Read the model definition and answer for the solid it produces. Units are mm, in the model's axes. Face numbers are marked on the shaded views. A direction names the side the tool comes from. Round coordinates to 2 decimals unless told otherwise and drop trailing zeros. Order: outer loops, then holes, each group sorted by start corner. A loop starts at its lowest first (then second) coordinate and runs counter-clockwise, first axis right, second up. Notation, with made-up numbers: (-31.75, -5.75) -> (27.25, -5.75) arc R29 cw to (27.25, 24.25) -> close; hole circle Ø8 at (17, -8). An arc over 180 degrees is marked (long way). Use a Markdown table: item, result. Add a question column.
1. Section B-B, the plane x = 5 is taken. Give the vertices of the cut face in (y, z).
2. The mould has two halves that part along Y. Classify the marked faces 3, 4, 5 and 6: +Y half, -Y half, draft (parallel to the pull), parting line (faces both ways), or undercut.
3. For the marked faces 1 and 2, determine the directions among +Z, -Z, +X, -X, +Y, -Y from which every point of the face is accessible in a straight line to the end or side of a thin tool.
4. Given pin 1 (5 mm diameter, centred on x = 25, y = -5, fed in from -Z), flat-ended and moving along its own axis, determine where the tip first touches the part or whether it passes through.
5. Section C-C, the plane z = 2.55 is taken. Give the vertices of the cut face in (x, y).
6. Section D-D, the plane y = -30.5 is taken. Give the vertices of the cut face in (x, z).
7. Consider L1, parallel to Y at x = 25, z = 1.5; L2, parallel to X at y = -26.5, z = 2.35; L3, parallel to Y at x = 11, z = 0.3. Determine where each line is inside the solid, lowest interval first. Write a range as [from, to].
8. Section A-A, the plane y = -5 is taken. Give the vertices of the cut face in (x, z), then the cut area to 3 significant figures.
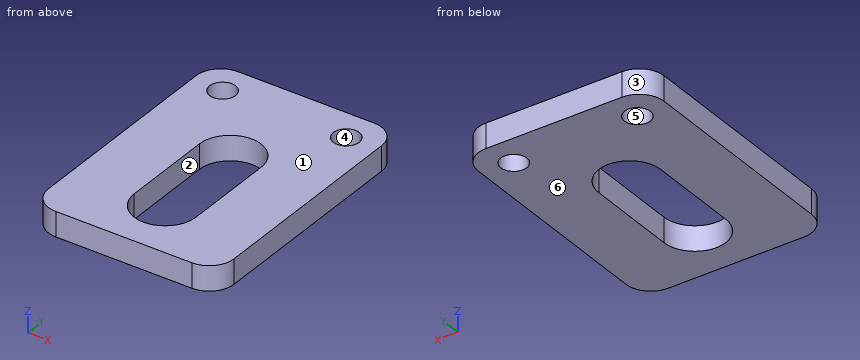
```python
from build123d import *

# Parameters (mm, degrees)
SKETCH_1_W          = 30
SKETCH_1_H          = 42
EXTRUDE_1_DEPTH     = 4
SKETCH_2_R          = 2.1
CUT_EXTRUDE_1_DEPTH = 52.768716422
FILLET_1_R          = 4


with BuildPart() as part:
    # 草图1 → 凸台-拉伸1 (new body)
    with BuildSketch(Plane.XY):
        with Locations((15, -21)):
            Rectangle(SKETCH_1_W, SKETCH_1_H)
    extrude(amount=EXTRUDE_1_DEPTH)

    # 草图2 → 切除-拉伸1 (cut, through all)
    with BuildSketch(Plane.XY.offset(4)):
        with Locations((5, -5)):
            Circle(SKETCH_2_R)
        with Locations((25, -5)):
            Circle(SKETCH_2_R)
        with BuildLine():
            Line((20, -17.5), (20, -32.5))
            ThreePointArc((20, -32.5), (15, -37.5), (10, -32.5))
            Line((10, -32.5), (10, -17.5))
            ThreePointArc((10, -17.5), (15, -12.5), (20, -17.5))
        make_face()
    extrude(amount=-CUT_EXTRUDE_1_DEPTH, mode=Mode.SUBTRACT)

    # 圆角1
    fillet_1_edges = [part.edges().sort_by_distance(p)[0] for p in [
        (0, 0, 2),
        (30, 0, 2),
        (30, -42, 2),
        (0, -42, 2),
    ]]
    fillet(fillet_1_edges, radius=FILLET_1_R)


solid = part.part
```
Verdict:
| question | item | result |
|---|---|---|
| 1 | outline | (-42, 0) -> (-7.1, 0) -> (-7.1, 4) -> (-42, 4) -> close; (-2.9, 0) -> (0, 0) -> (0, 4) -> (-2.9, 4) -> close |
| 2 | face 3 | +Y half |
| 2 | face 4 | undercut |
| 2 | face 5 | undercut |
| 2 | face 6 | draft |
| 3 | face 1 | +Z, +X, -X, +Y, -Y |
| 3 | face 2 | +Z, -Z |
| 4 | pin 1 | stops at z = 0 |
| 5 | outline | (0, -38) arc R4 ccw to (4, -42) -> (26, -42) arc R4 ccw to (30, -38) -> (30, -4) arc R4 ccw to (26, 0) -> (4, 0) arc R4 ccw to (0, -4) -> close; hole circle Ø4.2 at (5, -5); hole (10, -32.5) arc R5 ccw to (20, -32.5) -> (20, -17.5) arc R5 ccw to (10, -17.5) -> close; hole circle Ø4.2 at (25, -5) |
| 6 | outline | (0, 0) -> (10, 0) -> (10, 4) -> (0, 4) -> close; (20, 0) -> (30, 0) -> (30, 4) -> (20, 4) -> close |
| 7 | L1 | y = [-42, -7.1], [-2.9, 0] |
| 7 | L2 | x = [0, 10], [20, 30] |
| 7 | L3 | y = [-42, -35.5], [-14.5, 0] |
| 8 | outline | (0, 0) -> (2.9, 0) -> (2.9, 4) -> (0, 4) -> close; (7.1, 0) -> (22.9, 0) -> (22.9, 4) -> (7.1, 4) -> close; (27.1, 0) -> (30, 0) -> (30, 4) -> (27.1, 4) -> close |
| 8 | area | 86.4 mm2 |
